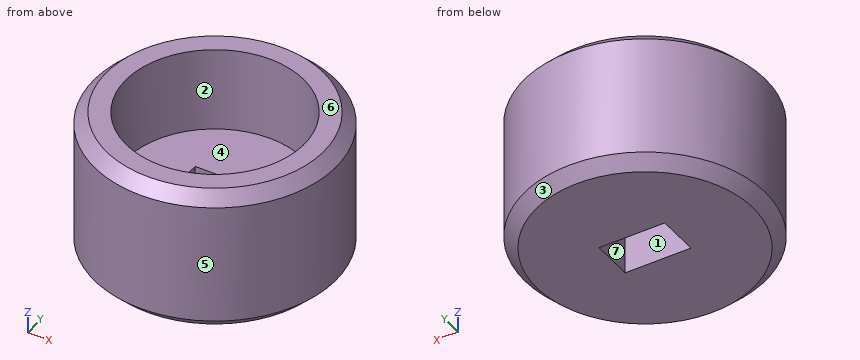
from build123d import *

# Parameters (mm, degrees)
SKETCH001_R     = 10
PAD_DEPTH       = 6
SKETCH_W        = 5.5
SKETCH_H        = 3.5
POCKET_DEPTH    = 12.001
SKETCH002_R     = 7.375
POCKET001_DEPTH = 7
CHAMFER_SIZE    = 1


with BuildPart() as part:
    # Sketch001 → Pad (new body, symmetric)
    with BuildSketch(Plane.XY):
        Circle(SKETCH001_R)
    extrude(amount=PAD_DEPTH, both=True)

    # Sketch → Pocket (cut, through all)
    with BuildSketch(Plane(origin=(0, 0, -6), x_dir=(1, 0, 0), z_dir=(0, 0, -1))):
        Rectangle(SKETCH_W, SKETCH_H)
    extrude(amount=-POCKET_DEPTH, mode=Mode.SUBTRACT)

    # Sketch002 → Pocket001 (cut)
    with BuildSketch(Plane.XY.offset(6)):
        Circle(SKETCH002_R)
    extrude(amount=-POCKET001_DEPTH, mode=Mode.SUBTRACT)

    # Chamfer
    chamfer_edges = [part.edges().sort_by_distance(p)[0] for p in [
        (-10, 0, 6),
        (-10, 0, -6),
    ]]
    chamfer(chamfer_edges, length=CHAMFER_SIZE)


solid = part.part
Geometry: final body of the model. Coordinates: model frame, mm. Face numbers are marked on the shaded views. A direction names the side the tool comes from. Coordinates: 2 decimals unless noted, no trailing zeros. Loops run counter-clockwise (first coordinate to the right, second up) from the corner with the lowest first, then second, coordinate; pieces in that order, holes last. Notation, with made-up numbers: (-25.5, 19) - (17.5, 19) arc R6 cw to (17.5, 24) - close; hole circle Ø4 at (-2.5, 85). An arc over 180 degrees is marked (long way). One line per question, with ' | ' between items. Start each with the question number.
(1) Reachability of the marked faces 1, 2 and 3 from +Z, -Z, +X, -X, +Y, -Y: full face, straight path, thin tool, end or side. Return the list, or none.
(2) Cut plane D-D on z = 1. Output: boundary loops of the cut face in (x, y) (3 decimals), and give its area (3 significant figures).
(3) Draft query along X for the marked faces 4, 5, 6 and 7. Return one class per face: +X half, -X half, draft (parallel to the pull), parting line (faces both ways), or undercut.
(4) Ray query, L1, parallel to Y at x = 0, z = 3.75 (3 decimals); L2, parallel to Y at x = 1.5, z = 5.75; L3, parallel to Z at x = 2.5, y = 3.75. Return the intervals inside material, ascending. Write a range as from..to.
(5) First-contact query: pin 1 (4 mm diameter, centred on x = -3, z = -2.5, fed in from -Y); pin 2 (3 mm diameter, centred on x = -3, z = -1.5, fed in from +Y); pin 3 (1 mm diameter, centred on x = 3, z = -2, fed in from -Y). Flat tips, straight axial feed; report the tip coordinate or a pass-through.
(6) Cut plane A-A on x = 0. Output: boundary loops of the cut face in (y, z) (3 decimals).
(7) Cut plane B-B on y = 0. Output: boundary loops of the cut face in (x, z) (3 decimals), and give its area (3 significant figures).
(8) Cut plane C-C on z = -3.5. Output: boundary loops of the cut face in (x, y).
Here are the results:
1) face 1: +Z, -Z | face 2: +Z | face 3: -Z
2) outline: circle Ø20 at (0, 0); hole circle Ø14.75 at (0, 0) | area: 143 mm²
3) face 4: undercut | face 5: parting line | face 6: draft | face 7: undercut
4) L1: -10..-7.375, 7.375..10 | L2: -9.13..-7.22, 7.22..9.13 | L3: -6..-1
5) pin 1: y = -9.95 | pin 2: y = 9.89 | pin 3: y = -9.68
6) outline: (-10, -5) - (-9, -6) - (-1.75, -6) - (-1.75, -1) - (-7.375, -1) - (-7.375, 6) - (-9, 6) - (-10, 5) - close; (1.75, -6) - (9, -6) - (10, -5) - (10, 5) - (9, 6) - (7.375, 6) - (7.375, -1) - (1.75, -1) - close
7) outline: (-10, -5) - (-9, -6) - (-2.75, -6) - (-2.75, -1) - (-7.375, -1) - (-7.375, 6) - (-9, 6) - (-10, 5) - close; (2.75, -6) - (9, -6) - (10, -5) - (10, 5) - (9, 6) - (7.375, 6) - (7.375, -1) - (2.75, -1) - close | area: 107 mm²
8) outline: circle Ø20 at (0, 0); hole (-2.75, -1.75) - (2.75, -1.75) - (2.75, 1.75) - (-2.75, 1.75) - close
